```python
from build123d import *

# Parameters (mm, degrees)
F1_DEPTH  = 25.4
F3_DEPTH  = 6.35
F5_DEPTH  = 7.9375
F6_W      = 12.7
F6_H      = 1.905
F7_DEPTH  = 6.858
F8_W      = 1.190625
F8_H      = 1.905
F9_DEPTH  = 12.7
F11_DEPTH = 25.4
F12_W     = 15.08125
F12_H     = 12.7
F13_DEPTH = 5.3578125
F14_R     = 2.5796875
F15_DEPTH = 25.4
F18_DEPTH = 25.4
F19_W     = 25.003125
F19_H     = 9.921875
F20_DEPTH = 4.5640625
F21_R     = 2.54
F22_R     = 2.54
F23_R     = 5.08


with BuildPart() as f1:
    # F0 (on Front) → F1 (new body)
    with BuildSketch(Plane.XZ):
        with BuildLine():
            ThreePointArc((9.525, 43.5474833257), (34.7253859158, 27.9509660298), (44.577, 0))
            ThreePointArc((44.577, 0), (-27.9509660298, -34.7253859158), (-9.525, 43.5474833257))
            Line((-9.525, 43.5474833257), (-9.525, 49.8990418245))
            ThreePointArc((-9.525, 49.8990418245), (-32.3787739113, -39.1440289189), (50.8, 0))
            ThreePointArc((50.8, 0), (39.1440289189, 32.3787739113), (9.525, 49.8990418245))
            Line((9.525, 49.8990418245), (9.525, 43.5474833257))
        make_face()
        with BuildLine():
            ThreePointArc((-9.525, 43.5474833257), (0, 44.577), (9.525, 43.5474833257))
            Line((9.525, 43.5474833257), (9.525, 49.8990418245))
            ThreePointArc((9.525, 49.8990418245), (0, 50.8), (-9.525, 49.8990418245))
            Line((-9.525, 49.8990418245), (-9.525, 43.5474833257))
        make_face()
        with BuildLine():
            ThreePointArc((-9.525, 49.8990418245), (0, 50.8), (9.525, 49.8990418245))
            Line((9.525, 49.8990418245), (9.525, 63.5))
            Line((9.525, 63.5), (-9.525, 63.5))
            Line((-9.525, 63.5), (-9.525, 49.8990418245))
        make_face()
    extrude(amount=F1_DEPTH)

    # F2 (on face) → F3 (cut)
    with BuildSketch(Plane.XZ.offset(25.4)):
        with BuildLine():
            ThreePointArc((0.8929687032, 50.3226047716), (2.6789062266, 50.322604731), (3.571875, 51.8692719891))
            ThreePointArc((3.571875, 51.8692719891), (1.7859375, 53.6552094891), (0, 51.8692719891))
            ThreePointArc((0, 51.8692719891), (0.2392702419, 50.9763032626), (0.8929687032, 50.3226047716))
        make_face()
        with BuildLine():
            ThreePointArc((-0.8929687383, 50.3226047513), (-0.2392702521, 50.976303245), (0, 51.8692719891))
            ThreePointArc((0, 51.8692719891), (-3.3326047479, 52.7622407333), (-0.8929687383, 50.3226047513))
        make_face()
        with BuildLine():
            ThreePointArc((0.8929687032, 50.3226047716), (0.2392702419, 50.9763032626), (0, 51.8692719891))
            ThreePointArc((0, 51.8692719891), (-0.2392702521, 50.976303245), (-0.8929687383, 50.3226047513))
            ThreePointArc((-0.8929687383, 50.3226047513), (-2.03e-08, 50.561875), (0.8929687032, 50.3226047716))
        make_face()
        with BuildLine():
            ThreePointArc((1.7859375, 48.7759375), (1.546667231, 49.6689062734), (0.8929687032, 50.3226047716))
            ThreePointArc((0.8929687032, 50.3226047716), (-2.03e-08, 50.561875), (-0.8929687383, 50.3226047513))
            ThreePointArc((-0.8929687383, 50.3226047513), (-0.8929687558, 47.2292702588), (1.7859375, 48.7759375))
        make_face()
    extrude(amount=-F3_DEPTH, mode=Mode.SUBTRACT)

    # F4 (on face) → F5 (cut)
    with BuildSketch(Plane.XZ.offset(25.4)):
        Polygon((-6.9453125, 60.6226043245), (-6.9453125, 54.4710418245), (6.9453125, 54.4710418245), (6.9453125, 60.6226043245), align=None)
    extrude(amount=-F5_DEPTH, mode=Mode.SUBTRACT)

    # F6 (on face) → F7 (cut)
    with BuildSketch(Plane.XY.offset(63.5)):
        with Locations((0, -15.71625)):
            Rectangle(F6_W, F6_H)
    extrude(amount=-F7_DEPTH, mode=Mode.SUBTRACT)

    # F8 (on face) → F9 (join)
    with BuildSketch(Plane.XY.offset(63.5)):
        with Locations((2.778125, -15.71625)):
            Rectangle(F8_W, F8_H)
        with Locations((-2.778125, -15.71625)):
            Rectangle(F8_W, F8_H)
    extrude(amount=-F9_DEPTH)

    # F10 (on Front) → F11 (join)
    with BuildSketch(Plane.XZ):
        with BuildLine():
            Line((-30.48, -65.0875), (30.48, -65.0875))
            Line((30.48, -65.0875), (30.48, -40.64))
            ThreePointArc((30.48, -40.64), (0, -50.8), (-30.48, -40.64))
            Line((-30.48, -40.64), (-30.48, -65.0875))
        make_face()
    extrude(amount=F11_DEPTH)

    # F12 (on face) → F13 (cut)
    with BuildSketch(Plane(origin=(0, 0, -65.0875), x_dir=(1, 0, 0), z_dir=(0, 0, -1))):
        with Locations((20.0421875, 12.7)):
            Rectangle(F12_W, F12_H)
        with Locations((-20.0421875, 12.7)):
            Rectangle(F12_W, F12_H)
    extrude(amount=-F13_DEPTH, mode=Mode.SUBTRACT)

    # F14 (on face) → F15 (cut)
    with BuildSketch(Plane(origin=(0, 0, -59.7296875), x_dir=(1, 0, 0), z_dir=(0, 0, -1))):
        with Locations((21.2328125, 12.7)):
            Circle(F14_R)
        with Locations((-21.2328125, 12.7)):
            Circle(F14_R)
    extrude(amount=-F15_DEPTH, mode=Mode.SUBTRACT)

    # F17 (on offset) → F18 (cut)
    with BuildSketch(Plane.XY.offset(-48.26)):
        Polygon((18.9414536192, -16.66875), (23.5241713808, -16.66875), (25.8155302617, -12.7), (23.5241713808, -8.73125), (18.9414536192, -8.73125), (16.6500947383, -12.7), align=None)
        Polygon((-25.8155302617, -12.7), (-23.5241713808, -16.66875), (-18.9414536192, -16.66875), (-16.6500947383, -12.7), (-18.9414536192, -8.73125), (-23.5241713808, -8.73125), align=None)
    extrude(amount=F18_DEPTH, mode=Mode.SUBTRACT)

    # F19 (on face) → F20 (cut)
    with BuildSketch(Plane(origin=(0, 0, -65.0875), x_dir=(1, 0, 0), z_dir=(0, 0, -1))):
        with Locations((0, 12.7)):
            Rectangle(F19_W, F19_H)
    extrude(amount=-F20_DEPTH, mode=Mode.SUBTRACT)

    # F21
    f21_edges = [f1.edges().sort_by_distance(p)[0] for p in [
        (-30.48, -12.7, -65.0875),
        (30.48, -12.7, -65.0875),
    ]]
    fillet(f21_edges, radius=F21_R)

    # F22
    f22_edges = [f1.edges().sort_by_distance(p)[0] for p in [
        (-9.525, -12.7, 63.5),
        (9.525, -12.7, 63.5),
    ]]
    fillet(f22_edges, radius=F22_R)

    # F23
    f23_edges = [f1.edges().sort_by_distance(p)[0] for p in [
        (9.525, -12.7, 49.899042),
        (-9.525, -12.7, 49.899042),
        (30.48, -12.7, -40.64),
        (-30.48, -12.7, -40.64),
    ]]
    fillet(f23_edges, radius=F23_R)


solid = f1.part
```
Model file for the job. Use its own axes, mm. A direction names the side the tool comes from. Give positions to 0.01 mm unless a question says otherwise; leave off trailing zeros. Write each loop counter-clockwise with the first axis right and the second up, starting at its lowest first coordinate (ties: lowest second). Pieces come first, ordered by that corner, then holes. Notation, with made-up numbers: M -17.75,59.5 L -9.75,59.5 A21 cw -9.75,88.5 Z; hole C -20,9.25 d3. An arc over 180 degrees is marked long. Use a Markdown table: item, result.
1) Drill centre lines: line 1 (X direction, y = -18.25, z = 0); line 2 (Z direction, x = 0, y = -12.75); line 3 (Z direction, x = -19, y = -3.5). Where is each one in solid material? Low to high. Write a range as from..to.
Responses:
| item | result |
|---|---|
| line 1 | x = -50.8..-44.58, 44.58..50.8 |
| line 2 | z = -60.52..-44.58, 44.58..63.5 |
| line 3 | z = -65.09..-40.33, 40.33..47.11 |
2) Cut at B-B (y = -21). List the corners of the cut face in (x, z) (1 decimal).
Responses:
| item | result |
|---|---|
| outline | M -32.3,-39.2 A5.1 cw -30.5,-43.1 L -30.5,-62.5 A2.5 ccw -27.9,-65.1 L 27.9,-65.1 A2.5 ccw 30.5,-62.5 L 30.5,-43.1 A5.1 cw 32.3,-39.2 A50.8 ccw 13.3,49 A5.1 cw 9.5,53.9 L 9.5,61 A2.5 ccw 7,63.5 L -7,63.5 A2.5 ccw -9.5,61 L -9.5,53.9 A5.1 cw -13.3,49 A50.8 ccw Z; hole C 0,0 d89.2; hole M -6.9,54.5 L 6.9,54.5 L 6.9,60.6 L -6.9,60.6 Z; hole M -0.9,50.3 A1.8 ccw long 0.9,50.3 A1.8 ccw long 0,51.9 A1.8 ccw long Z |
3) Cut at C-C (x = -5). List the corners of the cut face in (y, z), and give its area (3 significant figures).
Responses:
| item | result |
|---|---|
| outline | M -25.4,-65.09 L -17.66,-65.09 L -17.66,-60.52 L -7.74,-60.52 L -7.74,-65.09 L 0,-65.09 L 0,-44.3 L -25.4,-44.3 Z; M -25.4,44.3 L 0,44.3 L 0,63.5 L -14.76,63.5 L -14.76,56.64 L -16.67,56.64 L -16.67,63.5 L -25.4,63.5 L -25.4,60.62 L -17.46,60.62 L -17.46,54.47 L -25.4,54.47 Z |
| area | 909 mm2 |
4) Pull direction Y, two halves, no side cores. Call faces 1 (the flat face through (11.1, -25.4, -43.4)), 2 (the cylindrical face through (23.616, -11.712, -54.075)), 3 (the cylindrical face through (-49.486, -12.522, 11.481)), 4 (the flat face through (-11.5, 0, -43.4)): +Y half, -Y half, draft (parallel to the pull), parting line (faces both ways), or undercut.
Responses:
| item | result |
|---|---|
| face 1 | -Y half |
| face 2 | undercut |
| face 3 | draft |
| face 4 | +Y half |
5) Tool access for faces 5 (the flat face through (24, -13, -48.26)), 6 (the cylindrical face through (-3.3, -22.27, 52.82)), 7 (the flat face through (-5, -16.669, 60)), 8 (the flat face through (-18, -13, -59.73)): list every direction of +Z, -Z, +X, -X, +Y, -Y with a clear straight run to the whole face (end or side of a thin tool).
Responses:
| item | result |
|---|---|
| face 5 | none |
| face 6 | -Y |
| face 7 | +Z |
| face 8 | -Z |
6) Cut at A-A (z = 0). List the corners of the cut face in (x, y).
Responses:
| item | result |
|---|---|
| outline | M -50.8,-25.4 L -44.58,-25.4 L -44.58,0 L -50.8,0 Z; M 44.58,-25.4 L 50.8,-25.4 L 50.8,0 L 44.58,0 Z |
7) Pin check, flat tips, straight feed: pin 1 (2.5 mm diameter, centred on x = 19.5, z = -62.5, fed in from +Y); pin 2 (6 mm diameter, centred on y = -12.5, z = -55.5, fed in from +X); pin 3 (0.6 mm diameter, centred on y = -15.5, z = 61, fed in from -X) (3 decimals); pin 4 (5 mm diameter, centred on x = 10.5, y = -4.5, fed in from +Z). Stop position of each tip, or through.
Responses:
| item | result |
|---|---|
| pin 1 | stops at y = 0 |
| pin 2 | stops at x = 30.48 |
| pin 3 | stops at x = -9.525 |
| pin 4 | stops at z = 63.29 |
